from build123d import *

# Parameters (mm, degrees)
SKETCH1_W            = 17
SKETCH1_H            = 35
BOSS_EXTRUDE1_DEPTH  = 3
M3_CLEARANCE_HOLE1_D = 3.6
SKETCH5_W            = 9.7
SKETCH5_H            = 6.05
BOSS_EXTRUDE2_DEPTH  = 12
CUT_EXTRUDE1_DEPTH   = 12
BOSS_EXTRUDE3_DEPTH  = 12
SKETCH8_W            = 17
SKETCH8_H            = 15
BOSS_EXTRUDE4_DEPTH  = 30
CUT_EXTRUDE2_START   = -15
CUT_EXTRUDE2_DEPTH   = 15


# Read off the part's stored shape, not the designer's step: Cut-Extrude2
with BuildPart() as part:
    # Sketch1 → Boss-Extrude1 (new body)
    with BuildSketch(Plane(origin=(0, 0, 0), x_dir=(1, 0, 0), z_dir=(0, 1, 0))):
        with Locations((-3.5, 0)):
            Rectangle(SKETCH1_W, SKETCH1_H)
    extrude(amount=BOSS_EXTRUDE1_DEPTH)

    # M3 Clearance Hole1 (through all)
    with Locations(Plane(origin=(0, 0, 0), x_dir=(-1, 0, 0), z_dir=(0, -1, 0))):
        with Locations((2, 13.5), (2, -13.5)):
            Hole(M3_CLEARANCE_HOLE1_D / 2)

    # Sketch5 → Boss-Extrude2 (add)
    with BuildSketch(Plane(origin=(0, 3, 0), x_dir=(1, 0, 0), z_dir=(0, 1, 0))):
        with Locations((0.15, -14.475)):
            Rectangle(SKETCH5_W, SKETCH5_H)
        with Locations((0.15, 14.475)):
            Rectangle(SKETCH5_W, SKETCH5_H)
    extrude(amount=BOSS_EXTRUDE2_DEPTH)

    # Sketch6 → Cut-Extrude1 (cut)
    with BuildSketch(Plane(origin=(0, 15, 0), x_dir=(1, 0, 0), z_dir=(0, 1, 0))):
        with BuildLine():
            Line((-3.8, -13.5), (-3.8, 13.5))
            ThreePointArc((-3.8, 13.5), (-2, 15.3), (-0.2, 13.5))
            Line((-0.2, 13.5), (-0.2, -13.5))
            ThreePointArc((-0.2, -13.5), (-2, -15.3), (-3.8, -13.5))
        make_face()
    extrude(amount=-CUT_EXTRUDE1_DEPTH, mode=Mode.SUBTRACT)

    # Sketch7 → Boss-Extrude3 (add)
    with BuildSketch(Plane(origin=(0, 3, 0), x_dir=(1, 0, 0), z_dir=(0, 1, 0))):
        Polygon((-12, -17.5), (-4.7, -17.5), (-4.7, -16.25), (-7.5, -16.25), (-7.5, -11.45), (-12, -11.45), align=None)
        Polygon((-12, 17.5), (-4.7, 17.5), (-4.7, 16.25), (-7.5, 16.25), (-7.5, 11.45), (-12, 11.45), align=None)
    extrude(amount=BOSS_EXTRUDE3_DEPTH)

    # Sketch8 → Boss-Extrude4 (add)
    with BuildSketch(Plane(origin=(0, 0, -17.5), x_dir=(-1, 0, 0), z_dir=(0, 0, -1))):
        with Locations((3.5, 7.5)):
            Rectangle(SKETCH8_W, SKETCH8_H)
    extrude(amount=BOSS_EXTRUDE4_DEPTH)

    # Cut-Extrude2 outline → Cut-Extrude2 (cut)
    with BuildSketch(Plane(origin=(0, 15, 0), x_dir=(1, 0, 0), z_dir=(0, 1, 0)).offset(CUT_EXTRUDE2_START)):
        with BuildLine():
            ThreePointArc((-12, 16.695382119), (-3.71171241, 20.348605395), (5, 22.828084846))
            Line((5, 22.828084846), (5, 47.5))
            Line((5, 47.5), (-12, 47.5))
            Line((-12, 47.5), (-12, 16.695382119))
        make_face()
    extrude(amount=CUT_EXTRUDE2_DEPTH, mode=Mode.SUBTRACT)


solid = part.part
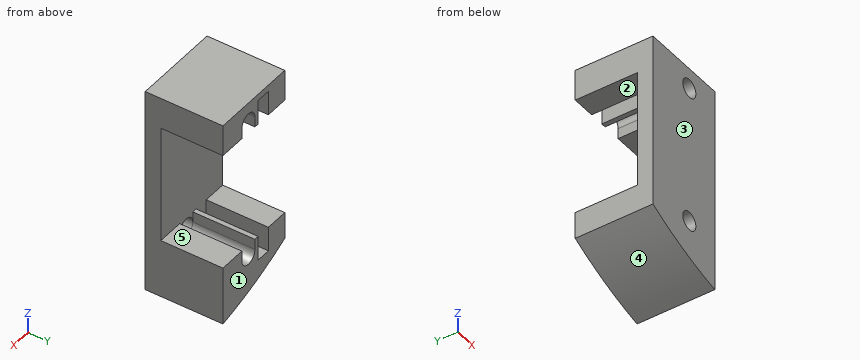
The model under review builds one solid part; all positions refer to its coordinate system, in mm. Face numbers are marked on the shaded views. A direction names the side the tool comes from. Give positions to 0.01 mm unless a question says otherwise; leave off trailing zeros. Write each loop counter-clockwise with the first axis right and the second up, starting at its lowest first coordinate (ties: lowest second). Pieces come first, ordered by that corner, then holes.
1. Tool access review of the marked faces 1 and 2: name each direction out of +Z, -Z, +X, -X, +Y, -Y from which nothing blocks a thin tool from reaching the whole face with its end or side.
2. For P1, Ø2, axis at x = -6, y = 6.5, coming from the -Z side; P2, Ø1, axis at x = -4.5, y = 8.5, coming from the -Z side; P3, Ø5, axis at x = -5.5, z = -3.5, coming from the +Y side, all flat-tipped, find the tip position at first contact; note any pin that passes through.
3. Wall thickness on L1, parallel to X at y = 9, z = 13.5; L2, parallel to Z at x = -2, y = 2.1; L3, parallel to X at y = 2.4, z = -13.5: over which ranges is each line inside the solid? List them lowest first.
4. Draft analysis for pull direction Z (two halves, no side actions). For the marked faces 3, 4 and 5, state which applies: +Z half, -Z half, draft (parallel to the pull), parting line (faces both ways), or undercut.
5. Add section B-B, the plane x = -1. Write out the cut boundary in (y, z).
6. Add section D-D, the plane x = -6.5. Write out the cut boundary in (y, z), plus the area to 3 significant figures.
7. Add section C-C, the plane z = 12.5. Write out the cut boundary in (x, y), plus the area to 3 significant figures.
8. Add section A-A, the plane y = 4.75. Write out the cut boundary in (x, z).
Worked answers:
1. face 1: +Z, -Z, +X, -X, +Y
1. face 2: +X, -X, +Y
2. P1: stops at z = -19.87
2. P2: stops at z = -20.24
2. P3: stops at y = 3
3. L1: x = -12 to -7.5, -4.7 to -3.8, -0.2 to 5
3. L2: z = -20.94 to -15.3, -11.7 to 11.7, 15.3 to 17.5
3. L3: x = -12 to -3.8, -0.2 to 5
4. face 3: draft
4. face 4: -Z half
4. face 5: undercut
5. outline: (0, -21.26) - (15, -21.26) - (15, -15) - (0, -15) - close; (0, -12) - (3, -12) - (3, 12) - (0, 12) - close; (0, 15) - (15, 15) - (15, 17.5) - (0, 17.5) - close
6. outline: (0, -19.27) - (15, -19.27) - (15, -16.25) - (3, -16.25) - (3, 16.25) - (15, 16.25) - (15, 17.5) - (0, 17.5) - close
6. area: 162 mm2
7. outline: (-12, 0) - (-3.5, 0) - (-3.5, 3) - (-3.8, 3) - (-3.8, 15) - (-4.7, 15) - (-4.7, 3) - (-7.5, 3) - (-7.5, 15) - (-12, 15) - close; (-0.5, 0) - (5, 0) - (5, 15) - (-0.2, 15) - (-0.2, 3) - (-0.5, 3) - close
7. area: 169 mm2
8. outline: (-12, -16.7) arc R65.75 ccw to (5, -22.83) - (5, -11.45) - (-0.2, -11.45) - (-0.2, -13.5) arc R1.8 cw to (-3.8, -13.5) - (-3.8, -11.45) - (-4.7, -11.45) - (-4.7, -16.25) - (-7.5, -16.25) - (-7.5, -11.45) - (-12, -11.45) - close; (-12, 11.45) - (-7.5, 11.45) - (-7.5, 16.25) - (-4.7, 16.25) - (-4.7, 11.45) - (-3.8, 11.45) - (-3.8, 13.5) arc R1.8 cw to (-0.2, 13.5) - (-0.2, 11.45) - (5, 11.45) - (5, 17.5) - (-12, 17.5) - close
